For this review, use the dimensioned drawing (mm, ordinates from the lowest corner) and the shaded views. Give positions to 0.01 mm unless a question says otherwise; leave off trailing zeros. Order: outer loops, then holes, each group sorted by start corner. A loop starts at its lowest first (then second) coordinate and runs counter-clockwise, first axis right, second up. Notation, with made-up numbers: (67, 70.25) - (74, 70.25) arc R22 ccw to (74, 90.25) - close; hole circle Ø7 at (-28, 73). An arc over 180 degrees is marked (long way). One line per item, written item: value.
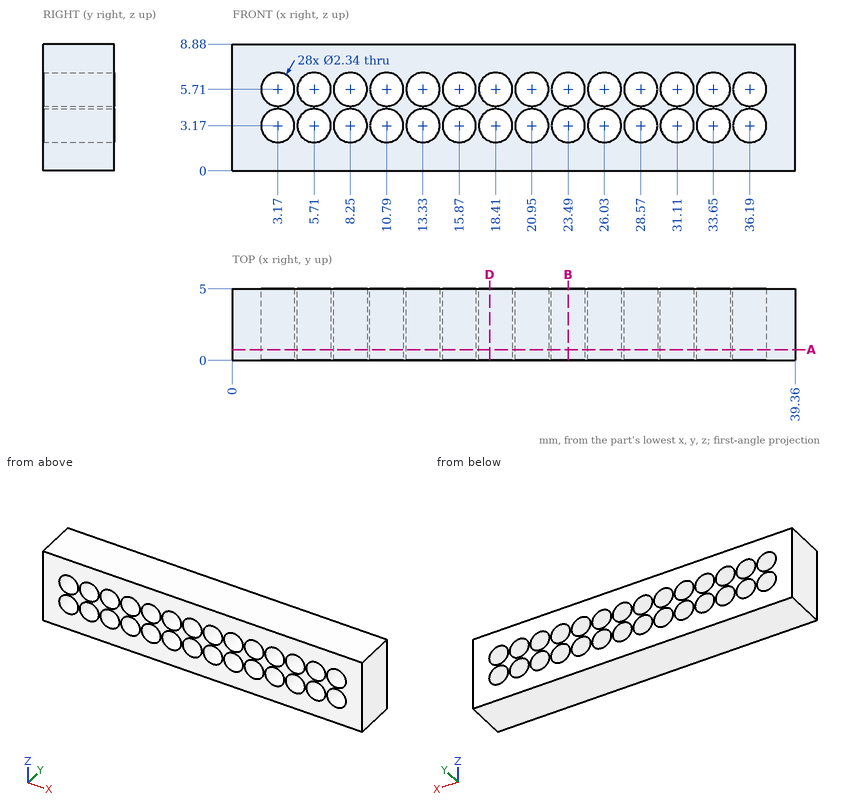
(1) Wall thickness on line 1 (Z direction, x = 3.17, y = 2.65); line 2 (Z direction, x = 36, y = 2.2): over which ranges is each line inside the solid? List them lowest first. Write a range as from..to.
Answers below:
line 1: z = 0..2, 4.34..4.54, 6.88..8.88
line 2: z = 0..2.02, 4.32..4.56, 6.86..8.88
(2) Take a section at D-D (x = 18). Write out the cut boundary in (y, z), then the cut area to 3 significant figures.
Answers below:
outline: (0, 0) - (5, 0) - (5, 2.07) - (0, 2.07) - close; (0, 4.27) - (5, 4.27) - (5, 4.61) - (0, 4.61) - close; (0, 6.81) - (5, 6.81) - (5, 8.88) - (0, 8.88) - close
area: 22.5 mm^2
(3) For P1, Ø2, axis at x = 13.33, z = 3.17, coming from the +Y side, flat-tipped, find the tip position at first contact; note if it passes through.
Answers below:
P1: passes through
(4) Take a section at B-B (x = 23.49). Write out the cut boundary in (y, z).
Answers below:
outline: (0, 0) - (5, 0) - (5, 2) - (0, 2) - close; (0, 4.34) - (5, 4.34) - (5, 4.54) - (0, 4.54) - close; (0, 6.88) - (5, 6.88) - (5, 8.88) - (0, 8.88) - close
(5) Take a section at A-A (y = 0.75). Give the number of separate pieces and of enclosed holes in the cut face, then the cut area to 3 significant figures.
Answers below:
separate pieces: 1
enclosed holes: 28
area: 229 mm^2
